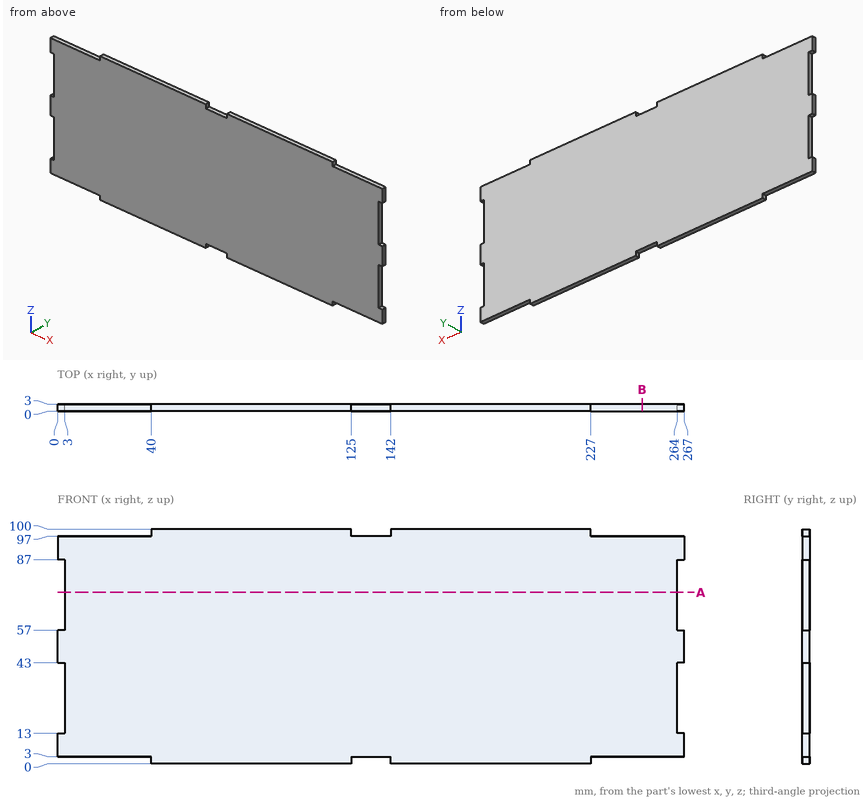
Here's the drawing with two shaded views (mm, measured from the low corner). I have some questions. Coordinates: 2 decimals unless noted, no trailing zeros. Order: outer loops, then holes, each group sorted by start corner. A loop starts at its lowest first (then second) coordinate and runs counter-clockwise, first axis right, second up.
Q1. Will these pins go through, and if not, where does the flat tip stop? pin 1 (0.9 mm diameter, centred on x = 266, y = 2, fed in from +Z); pin 2 (0.9 mm diameter, centred on y = 1.5, z = 22, fed in from +X); pin 3 (1 mm diameter, centred on x = 133.5, z = 11, fed in from -Y); pin 4 (0.9 mm diameter, centred on y = 1, z = 2, fed in from -X).
Q2. Suppose I cut it at B-B on x = 249. Please give me the cut outline in (y, z).
Q3. Suppose I cut it at A-A on z = 73. Please give me the cut outline in (x, y), and give its area (3 significant figures).
Q4. Please list where these lines run through material, in increasing order: L1, parallel to Z at x = 22, y = 2.05; L2, parallel to X at y = 1.75, z = 23.
Answer:
1. pin 1: stops at z = 97
1. pin 2: stops at x = 264
1. pin 3: stops at y = 0
1. pin 4: stops at x = 40
2. outline: (0, 3) - (3, 3) - (3, 97) - (0, 97) - close
3. outline: (3, 0) - (264, 0) - (264, 3) - (3, 3) - close
3. area: 783 mm2
4. L1: z = 3 to 97
4. L2: x = 3 to 264
